```python
from build123d import *

# Parameters (mm, degrees)
SKETCH1_W                 = 52
SKETCH1_H                 = 55
BOSS_EXTRUDE1_DEPTH       = 12.5
SKETCH2_R                 = 15
CUT_EXTRUDE2_DEPTH        = 13.5
F_5_0MM_DOWEL_HOLE1_D     = 5
F_5_0MM_DOWEL_HOLE1_DEPTH = 10
F_5_0MM_DOWEL_HOLE1_TIP   = 1.502151548


with BuildPart() as part:
    # Sketch1 → Boss-Extrude1 (new body)
    with BuildSketch(Plane.XY):
        with Locations((0, 27.5)):
            Rectangle(SKETCH1_W, SKETCH1_H)
    extrude(amount=BOSS_EXTRUDE1_DEPTH)

    # Sketch2 → Cut-Extrude2 (cut, through all)
    with BuildSketch(Plane.XY.offset(12.5)):
        with Locations((0, 27)):
            Circle(SKETCH2_R)
    extrude(amount=-CUT_EXTRUDE2_DEPTH, mode=Mode.SUBTRACT)

    # Ø5.0mm Dowel Hole1
    with Locations(Plane(origin=(0, 55, 0), x_dir=(1, 0, 0), z_dir=(0, 1, 0))):
        with Locations((-13.030851483, -6.229198753), (10.897813178, -6.229198753)):
            Hole(F_5_0MM_DOWEL_HOLE1_D / 2, depth=F_5_0MM_DOWEL_HOLE1_DEPTH)
            with Locations((0, 0, -(F_5_0MM_DOWEL_HOLE1_DEPTH + F_5_0MM_DOWEL_HOLE1_TIP / 2))):  # 118° drill point
                Cone(0, F_5_0MM_DOWEL_HOLE1_D / 2, F_5_0MM_DOWEL_HOLE1_TIP, mode=Mode.SUBTRACT)


solid = part.part
```
Input: part model. Units: mm. Frame: model coordinates. A direction names the side the tool comes from. Round coordinates to 2 decimals unless told otherwise and drop trailing zeros. Loops run counter-clockwise (first coordinate to the right, second up) from the corner with the lowest first, then second, coordinate; pieces in that order, holes last. Notation, with made-up numbers: M 47,78 L 69,78 A19 cw 69,84 Z; hole C -16.5,-10 d4. An arc over 180 degrees is marked long. Answer in a Markdown table with one row per item. Add a question column.
1. Section D-D (y = 46). Output: boundary loops of the cut face in (x, z).
2. Ray query, probe 1 along X at (y, z) = (20.5, 8.5); probe 2 along Y at (x, z) = (9, 1.5); probe 3 along Y at (x, z) = (-0.5, 3.5). Return the intervals inside material, ascending.
3. Mould query, pull axis Z, two halves, no side actions, for faces 1 (the face through (-12, 16, 12.5)), 2 (the face through (-26, 27, 6)), 3 (the face through (10.55, 43.76, 6.49)). Classes: released by +Z, released by -Z, zero draft, split by the parting line, or undercut.
4. Section B-B (x = 0). Output: boundary loops of the cut face in (y, z), and give its area (4 significant figures).
5. Section A-A (y = 27). Output: boundary loops of the cut face in (x, z).
6. Section C-C (z = 11). Output: boundary loops of the cut face in (x, y).
7. Set-up query: faces 4 (the face through (13.395, 49.93, 6.119)), 5 (the face through (26, 27, 6)). Return all of +Z, -Z, +X, -X, +Y, -Y with unobstructed straight access to the full face (end or side cutting, diameter ignored); none if empty.
Values follow:
| question | item | result |
|---|---|---|
| 1 | outline | M -26,0 L 26,0 L 26,12.5 L -26,12.5 Z; hole C -13.03,6.23 d5; hole C 10.9,6.23 d5 |
| 2 | probe 1 | -26 to -13.52, 13.52 to 26 |
| 2 | probe 2 | 0 to 15, 39 to 55 |
| 2 | probe 3 | 0 to 12.01, 41.99 to 55 |
| 3 | face 1 | released by +Z |
| 3 | face 2 | zero draft |
| 3 | face 3 | undercut |
| 4 | outline | M 0,0 L 12,0 L 12,12.5 L 0,12.5 Z; M 42,0 L 55,0 L 55,12.5 L 42,12.5 Z |
| 4 | area | 312.5 mm^2 |
| 5 | outline | M -26,0 L -15,0 L -15,12.5 L -26,12.5 Z; M 15,0 L 26,0 L 26,12.5 L 15,12.5 Z |
| 6 | outline | M -26,0 L 26,0 L 26,55 L -26,55 Z; hole C 0,27 d30 |
| 7 | face 4 | +Y |
| 7 | face 5 | +Z, -Z, +X, +Y, -Y |
